```python
from build123d import *

# Parameters (mm, degrees)
F0_R     = 10
F0_R_2   = 7.5
F1_DEPTH = 10


with BuildPart() as f1:
    # F0 (on Front) → F1 (new body)
    with BuildSketch(Plane.XZ):
        with BuildLine():
            Line((19.249851, 55.634453), (14.824665, 77.286766))
            ThreePointArc((14.824665, 77.286766), (0.358168, 89.995723), (-14.698586, 77.991918))
            Line((-14.698586, 77.991918), (-29.047106, 7.501041))
            Line((-29.047106, 7.501041), (-29.668046, 4.450513))
            ThreePointArc((-29.668046, 4.450513), (-12.900348, -27.084701), (22.151807, -20.231101))
            Line((22.151807, -20.231101), (84.240741, 39.498036))
            Line((84.240741, 39.498036), (87.778566, 42.9014))
            ThreePointArc((87.778566, 42.9014), (86.94615, 61.847062), (68.219281, 64.836271))
            Line((68.219281, 64.836271), (33.26649, 48.570462))
            ThreePointArc((33.26649, 48.570462), (24.54684, 48.70677), (19.249851, 55.634453))
        make_face()
        Circle(F0_R, mode=Mode.SUBTRACT)
        with Locations((0, 75)):
            Circle(F0_R_2, mode=Mode.SUBTRACT)
        with Locations((75.750642, 51.864047)):
            Circle(F0_R_2, mode=Mode.SUBTRACT)
        with BuildLine():
            Line((-29.668046, 4.450513), (-29.047106, 7.501041))
            ThreePointArc((-29.047106, 7.501041), (-29.397172, 5.983837), (-29.668046, 4.450513))
        make_face()
        with BuildLine():
            ThreePointArc((84.240741, 39.498036), (86.149827, 41.054007), (87.778566, 42.9014))
            Line((87.778566, 42.9014), (84.240741, 39.498036))
        make_face()
    extrude(amount=F1_DEPTH)


solid = f1.part
```
Source: CAD feature listing. Evaluate the final solid. Frame: model axes, mm. A direction names the side the tool comes from. Coordinates: 2 decimals unless noted, no trailing zeros. Write each loop counter-clockwise with the first axis right and the second up, starting at its lowest first coordinate (ties: lowest second). Pieces come first, ordered by that corner, then holes. Notation, with made-up numbers: (86, 58.25) -> (129, 58.25) arc R16 cw to (129, 86.25) -> close; hole circle Ø2 at (-35, 33.5). An arc over 180 degrees is marked (long way). Return JSON: item names as keys, results as strings. Group by question number.
1) Section query A-A, the plane x = 0. Return loops of the section in (y, z), plus the area to 3 significant figures.
2) Set-up query: faces 1 (the face through (50.99, -4.93, 56.82)), 2 (the face through (16, 0, 31)). Return all of +Z, -Z, +X, -X, +Y, -Y with unobstructed straight access to the full face (end or side cutting, diameter ignored); none if empty.
3) Mould query, pull axis X, two halves, no side actions, for faces 3 (the face through (3.461, -4.93, 68.346)), 4 (the face through (-2.17, -4.93, -9.76)), 5 (the face through (52.762, -4.93, 9.215)), 6 (the face through (-21.772, -4.93, 43.24)). Classes: +X half, -X half, draft (parallel to the pull), parting line (faces both ways), or undercut.
4) Section query D-D, the plane y = -3. Return loops of the section in (x, z), plus the area to 3 significant figures.
5) Section query B-B, the plane z = 75. Return loops of the section in (x, y), plus the area to 3 significant figures.
6) Contact query for flat-ended pins moving along their axis: P1, Ø16, axis at x = 0, z = 0, coming from the +Y side; P2, Ø5, axis at x = 39, y = -4.5, coming from the -Z side; P3, Ø1.5, axis at y = -4.5, z = -6.5, coming from the +X side; P4, Ø2, axis at x = 41, y = -6.5, coming from the +Z side. Output: stop coordinate, or through.
7) Ray query, line 1 along Z through (x, y) = (0, -2.25); line 2 along X through (y, z) = (-5.75, 55.5); line 3 along X through (y, z) = (-8, 52). Return the intervals inside material, ascending.
8) Section query C-C, the plane x = 71. Return loops of the section in (y, z).
From the geometry:
{
 "1": {"outline": "(-10, -30) -> (0, -30) -> (0, -10) -> (-10, -10) -> close; (-10, 10) -> (0, 10) -> (0, 67.5) -> (-10, 67.5) -> close; (-10, 82.5) -> (0, 82.5) -> (0, 90) -> (-10, 90) -> close", "area": "850 mm²"},
 "2": {"face 1": "+Z, +Y, -Y", "face 2": "+Z, -Z, +X, -X, +Y"},
 "3": {"face 3": "undercut", "face 4": "undercut", "face 5": "+X half", "face 6": "-X half"},
 "4": {"outline": "(-29.67, 4.45) arc R30 ccw to (22.15, -20.23) -> (84.24, 39.5) arc R15 ccw to (87.78, 42.9) arc R15 ccw to (68.22, 64.84) -> (33.27, 48.57) arc R10 cw to (19.25, 55.63) -> (14.82, 77.29) arc R15 ccw to (-14.7, 77.99) -> (-29.05, 7.5) arc R30 ccw to start; hole circle Ø20 at (0, 0); hole circle Ø15 at (0, 75); hole circle Ø15 at (75.75, 51.86)", "area": "7,360 mm²"},
 "5": {"outline": "(-15.31, -10) -> (-7.5, -10) -> (-7.5, 0) -> (-15.31, 0) -> close; (7.5, -10) -> (15.29, -10) -> (15.29, 0) -> (7.5, 0) -> close", "area": "156 mm²"},
 "6": {"P1": "through", "P2": "z = -6.43", "P3": "x = 37.21", "P4": "z = 52.63"},
 "7": {"line 1": "-30 to -10, 10 to 67.5, 82.5 to 90", "line 2": "-19.28 to 19.28, 48.16 to 69.19, 82.31 to 90.3", "line 3": "-19.99 to 20.79, 40.64 to 68.25, 83.25 to 90.75"},
 "8": {"outline": "(-10, 26.76) -> (0, 26.76) -> (0, 46.06) -> (-10, 46.06) -> close; (-10, 57.67) -> (0, 57.67) -> (0, 66.09) -> (-10, 66.09) -> close"}
}
